Check sheet for the modelled part. Datum: model origin and axes. Units: mm. Round coordinates to 2 decimals unless told otherwise and drop trailing zeros. Loops run counter-clockwise (first coordinate to the right, second up) from the corner with the lowest first, then second, coordinate; pieces in that order, holes last. Notation, with made-up numbers: (41, -9) - (79, -9) arc R29 ccw to (79, 28) - close; hole circle Ø7 at (-6, 84). An arc over 180 degrees is marked (long way). Answer in a Markdown table with one row per item. Add a question column.
(1) Gauge pin test, flat ends, axial feed: pin 1 (3 mm diameter, centred on y = 2.5, z = 158.5, fed in from -X); pin 2 (5 mm diameter, centred on y = 2, z = 277, fed in from -X); pin 3 (2 mm diameter, centred on y = -1.5, z = 80.5, fed in from +X). Record the tip position at first contact, or that the pin passes through.
(2) Cross-section at B-B on y = -2.25. Enter the section's corners in (x, z), then the cut area to 3 significant figures.
(3) Cross-section at A-A on x = 2.5. Enter the section's corners in (y, z), then the cut area to 3 significant figures.
(4) Cross-section at C-C on z = 236.5. Enter the section's corners in (x, y) (1 decimal), then the cut area to 3 significant figures.
(5) Thickness scan on line 1 along X through (y, z) = (-0.25, 19.5); line 2 along X through (y, z) = (0.75, 371.5); line 3 along Y through (x, z) = (-2.5, 27). Record the ranges inside material, lowest first.
Autodesk Inventor part; units mm, degrees
ref_plane "YZ Plane" through (0, 0, 0) normal (1, 0, 0) x (0, 1, 0)
ref_plane "XZ Plane" through (0, 0, 0) normal (0, 1, 0) x (-1, 0, 0)
ref_plane "XY Plane" through (0, 0, 0) normal (0, 0, 1) x (1, 0, 0)
sketch "Sketch1" plane through (0, 0, 0) normal (0, 0, 1) x (1, 0, 0)
  circle A0 centre (0, 0) radius 4.7625
  dimension "d0" = 9.525
extrude "Extrusion1" add sketch "Sketch1" along normal blind 397
sketch "Sketch2" plane through (0, 0, 397) normal (0, 0, 1) x (1, 0, 0)
  circle A0 centre (0, 0) radius 4.7625
  circle A1 centre (0, 0) radius 4
  dimension "d3" = 8
extrude "Extrusion2" add sketch "Sketch2" along normal blind 7 contours A1
sketch "Sketch3" plane through (0, 0, 0) normal (0, 0, -1) x (-1, 0, 0)
  circle A0 centre (0, 0) radius 4.7625
  circle A1 centre (0, 0) radius 4
  dimension "d6" = 8
extrude "Extrusion3" add sketch "Sketch3" along normal blind 30 contours A1
thread "Thread1"
properties part number "x_acme_upgrade"
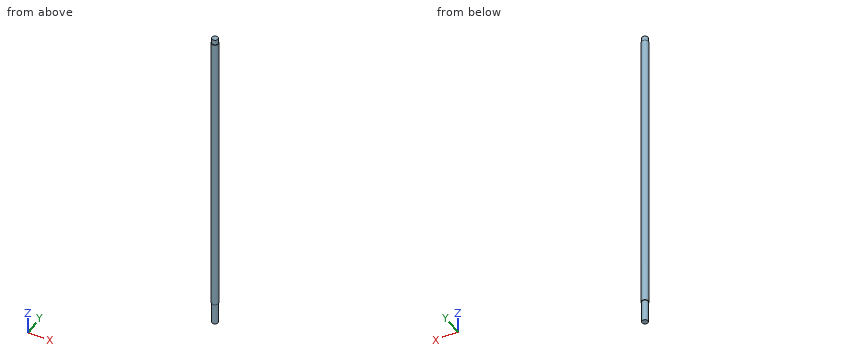
Answers:
| question | item | result |
|---|---|---|
| 1 | pin 1 | stops at x = -4.66 |
| 1 | pin 2 | stops at x = -4.76 |
| 1 | pin 3 | stops at x = 4.74 |
| 2 | outline | (-4.2, 0) - (-3.31, 0) - (-3.31, -30) - (3.31, -30) - (3.31, 0) - (4.2, 0) - (4.2, 397) - (3.31, 397) - (3.31, 404) - (-3.31, 404) - (-3.31, 397) - (-4.2, 397) - close |
| 2 | area | 3,580 mm^2 |
| 3 | outline | (-4.05, 0) - (-3.12, 0) - (-3.12, -30) - (3.12, -30) - (3.12, 0) - (4.05, 0) - (4.05, 397) - (3.12, 397) - (3.12, 404) - (-3.12, 404) - (-3.12, 397) - (-4.05, 397) - close |
| 3 | area | 3,450 mm^2 |
| 4 | outline | circle Ø9.5 at (0, 0) |
| 4 | area | 71.3 mm^2 |
| 5 | line 1 | x = -4.76 to 4.76 |
| 5 | line 2 | x = -4.7 to 4.7 |
| 5 | line 3 | y = -4.05 to 4.05 |
